```python
from build123d import *

# Parameters (mm, degrees)
SKETCH1_W           = 10
SKETCH1_H           = 24
BODY_DEPTH          = 1.6
SKETCH2_W           = 10
SKETCH2_H           = 1.6
BOSS_EXTRUDE2_DEPTH = 1.6
FIN_CHAMFER_SIZE    = 1
SKETCH3_R           = 3.5
HOLE_DEPTH          = 4.2
FIN_DEPTH           = 17.604910635
SIDE_CUT_DEPTH      = 11
TOP_CUT_DEPTH       = 2.6


with BuildPart() as part:
    # Sketch1 → Body (new body)
    with BuildSketch(Plane.XY):
        with Locations((0, 7)):
            Rectangle(SKETCH1_W, SKETCH1_H)
    extrude(amount=BODY_DEPTH)

    # Sketch2 → Boss-Extrude2 (add)
    with BuildSketch(Plane(origin=(0, 0, 0), x_dir=(-1, 0, 0), z_dir=(0, 0, -1))):
        with Locations((0, 5.8)):
            Rectangle(SKETCH2_W, SKETCH2_H)
    extrude(amount=BOSS_EXTRUDE2_DEPTH)

    # Fin Chamfer
    fin_chamfer_edges = [part.edges().sort_by_distance(p)[0] for p in [
        (0, 6.6, -1.6),
    ]]
    chamfer(fin_chamfer_edges, length=FIN_CHAMFER_SIZE)

    # Sketch3 → Hole (cut, through all)
    with BuildSketch(Plane.XY.offset(1.6)):
        Circle(SKETCH3_R)
    extrude(amount=-HOLE_DEPTH, mode=Mode.SUBTRACT)

    # Sketch4 → Fin (add)
    with BuildSketch(Plane.XY.offset(1.6)):
        Polygon((-5, 19), (-5, 5.4), (-3.4, 5.4), (-3.4, 17.4), (3.4, 17.4), (3.4, 5.4), (5, 5.4), (5, 19), align=None)
    extrude(amount=FIN_DEPTH)

    # Sketch5 → Side Cut (cut, through all)
    with BuildSketch(Plane(origin=(5, 0, 0), x_dir=(0, 0, -1), z_dir=(1, 0, 0))):
        Polygon((-1.6, 5.4), (-9.6, 5.4), (-19.204910635, 5.4), (-19.204910635, 17.4), (-9.6, 17.4), align=None)
    extrude(amount=-SIDE_CUT_DEPTH, mode=Mode.SUBTRACT)

    # Sketch7 → Top Cut (cut, through all)
    with BuildSketch(Plane.XZ.offset(-17.4)):
        Polygon((-5, 19.204910635), (-5, 9.6), (0, 19.204910635), align=None)
        Polygon((5, 19.204910635), (0, 19.204910635), (5, 9.6), align=None)
    extrude(amount=-TOP_CUT_DEPTH, mode=Mode.SUBTRACT)


solid = part.part
```
Verification items for the finished model (mm, model axes). A direction names the side the tool comes from. Give positions to 0.01 mm unless a question says otherwise; leave off trailing zeros. Order: outer loops, then holes, each group sorted by start corner. A loop starts at its lowest first (then second) coordinate and runs counter-clockwise, first axis right, second up. Notation, with made-up numbers: M 63.5,75.25 L 97.5,75.25 A12 ccw 97.5,93.25 Z; hole C 49,-2 d4. An arc over 180 degrees is marked long. Return JSON: item names as keys, results as strings. Group by question number.
1) Section check C-C on z = 7. Record the cut outline in (x, y).
2) Section check B-B on x = 1. Record the cut outline in (y, z).
3) Go/stop test with flat-tipped pins: pin 1 Ø3 at (x, z) = (2, 11.5) entering from -Y; pin 2 Ø2.5 at (y, z) = (11, 7.5) entering from +X; pin 3 Ø0.5 at (x, z) = (0, -0.5) entering from +Y; pin 4 Ø2 at (x, z) = (-2.5, 2) entering from -Y. Record where each tip stops, or that it passes through.
4) Scan lines: line 1 (Y direction, x = 0, z = 1.3); line 2 (Y direction, x = -1.25, z = 3.25); line 3 (Z direction, x = 1.5, y = 4.75). Record each from-to range of solid material in increasing order.
5) Access from +Z, -Z, +X, -X, +Y, -Y to the whole of each face (thin tool, end or side, straight path). Record for faces 1 (the face through (0, 5, -1)), 2 (the face through (0, 13, 0)), 3 (the face through (3.4, 13, 5)).
6) Mould release check, pull along X, two halves, no side actions. Record for faces 4 (the face through (0, -5, 1)), 5 (the face through (-5, 10, 3)), 6 (the face through (3.233, -1.341, 0.811)): pulls with the +X half, pulls with the -X half, needs draft (parallel to the pull), parting line crosses it, or undercut.
7) Section check A-A on y = 0. Record the cut outline in (x, z), and give its area (3 significant figures).
8) Section check D-D on x = 4. Record the cut outline in (y, z), and give its area (3 significant figures).
Answer block:
{
 "1": {"outline": "M -5,13.5 L -3.4,13.5 L -3.4,17.4 L 3.4,17.4 L 3.4,13.5 L 5,13.5 L 5,19 L -5,19 Z"},
 "2": {"outline": "M -5,0 L -3.35,0 L -3.35,1.6 L -5,1.6 Z; M 3.35,0 L 5,0 L 5,-1.6 L 5.6,-1.6 L 6.6,-0.6 L 6.6,0 L 19,0 L 19,17.28 L 17.4,17.28 L 17.4,1.6 L 3.35,1.6 Z"},
 "3": {"pin 1": "stops at y = 17.4", "pin 2": "passes through", "pin 3": "stops at y = 6.6", "pin 4": "stops at y = -5"},
 "4": {"line 1": "y = -5 to -3.5, 3.5 to 19", "line 2": "y = 17.4 to 19", "line 3": "z = 0 to 1.6"},
 "5": {"face 1": "-Z, +X, -X, -Y", "face 2": "-Z, +X, -X, +Y", "face 3": "+Z, -Y"},
 "6": {"face 4": "needs draft", "face 5": "pulls with the -X half", "face 6": "undercut"},
 "7": {"outline": "M -5,0 L -3.5,0 L -3.5,1.6 L -5,1.6 Z; M 3.5,0 L 5,0 L 5,1.6 L 3.5,1.6 Z", "area": "4.80 mm^2"},
 "8": {"outline": "M -5,0 L 5,0 L 5,-1.6 L 5.6,-1.6 L 6.6,-0.6 L 6.6,0 L 19,0 L 19,11.52 L 17.4,11.52 L 17.4,9.6 L 5.4,1.6 L -5,1.6 Z", "area": "104 mm^2"}
}
